Read the model definition and answer for the solid it produces. Units are mm, in the model's axes. A direction names the side the tool comes from. Give positions to 0.01 mm unless a question says otherwise; leave off trailing zeros. Write each loop counter-clockwise with the first axis right and the second up, starting at its lowest first coordinate (ties: lowest second). Pieces come first, ordered by that corner, then holes. Notation, with made-up numbers: (74, 84.25) -> (116, 84.25) arc R21 cw to (116, 112.25) -> close; hole circle Ø7 at (23.5, 67.5). An arc over 180 degrees is marked (long way). Use a Markdown table: item, result.
from build123d import *

# Parameters (mm, degrees)
F0_R      = 6.445170834
F0_R_2    = 6.017003406
F1_DEPTH  = 25.4
F2_W      = 19.7259690613
F2_H      = 52.9098398983
F3_DEPTH  = 25.4
F5_W      = 19.7259690613
F5_H      = 13.0423298106
F6_DEPTH  = 25.4
F4_W      = 19.7259690613
F4_H      = 10.3523302823
F7_DEPTH  = 25.4
F8_R      = 9.8629845306
F9_DEPTH  = 13.208
F12_DEPTH = 10.414
F13_R     = 2.9880803611
F14_DEPTH = 25.4
F15_R     = 2.8379061559
F16_DEPTH = 25.4
F18_DEPTH = 50.8


with BuildPart() as f1:
    # F0 (on Top) → F1 (new body)
    with BuildSketch(Plane.XY):
        with BuildLine():
            Line((23.6895978451, -37.5162102282), (23.6895978451, 37.5162102282))
            ThreePointArc((23.6895978451, 37.5162102282), (0, 61.2058080733), (-23.6895978451, 37.5162102282))
            Line((-23.6895978451, 37.5162102282), (-23.6895978451, -37.5162102282))
            ThreePointArc((-23.6895978451, -37.5162102282), (0, -61.2058080733), (23.6895978451, -37.5162102282))
        make_face()
        with Locations((0, -37.5162102282)):
            Circle(F0_R, mode=Mode.SUBTRACT)
        with Locations((0, 37.5162102282)):
            Circle(F0_R_2, mode=Mode.SUBTRACT)
    extrude(amount=F1_DEPTH)

    # F2 (on face) → F3 (join)
    with BuildSketch(Plane.XY.offset(25.4)):
        Rectangle(F2_W, F2_H)
    extrude(amount=F3_DEPTH)

    # F5 (on face) → F6 (join)
    with BuildSketch(Plane.XY.offset(50.8)):
        with Locations((0, -19.9337550439)):
            Rectangle(F5_W, F5_H)
    extrude(amount=F6_DEPTH)

    # F4 (on face) → F7 (join)
    with BuildSketch(Plane.XY.offset(50.8)):
        with Locations((0, 21.278754808)):
            Rectangle(F4_W, F4_H)
    extrude(amount=F7_DEPTH)

    # F8 (on face) → F9 (join)
    with BuildSketch(Plane.XZ.offset(26.4549199492)):
        with Locations((0, 76.2)):
            Circle(F8_R)
    extrude(amount=-F9_DEPTH)

    # F11 (on face) → F12 (join)
    with BuildSketch(Plane(origin=(0, 26.4549199492, 0), x_dir=(-1, 0, 0), z_dir=(0, 1, 0))):
        with BuildLine():
            Line((-9.8629845306, 76.2), (9.8629845306, 76.2))
            ThreePointArc((9.8629845306, 76.2), (0, 86.0629845306), (-9.8629845306, 76.2))
        make_face()
    extrude(amount=-F12_DEPTH)

    # F13 (on face) → F14 (cut)
    with BuildSketch(Plane.XZ.offset(-16.0409199492)):
        with Locations((-1.1676928261, 80.6610658765)):
            Circle(F13_R)
    extrude(amount=-F14_DEPTH, mode=Mode.SUBTRACT)

    # F15 (on face) → F16 (cut)
    with BuildSketch(Plane(origin=(0, -13.2469199492, 0), x_dir=(-1, 0, 0), z_dir=(0, 1, 0))):
        with Locations((0, 81.546805799)):
            Circle(F15_R)
    extrude(amount=-F16_DEPTH, mode=Mode.SUBTRACT)

    # F17 (on face) → F18 (cut)
    with BuildSketch(Plane(origin=(-9.8629845306, 0, 0), x_dir=(0, -1, 0), z_dir=(-1, 0, 0))):
        with BuildLine():
            ThreePointArc((-16.1025896668, 50.8), (-1.3449997641, 36.0424100973), (13.4125901386, 50.8))
            Line((13.4125901386, 50.8), (-16.1025896668, 50.8))
        make_face()
    extrude(amount=-F18_DEPTH, mode=Mode.SUBTRACT)


solid = f1.part
Item 1: Straight lines are drawn through the part: line 1 along Y through (x, z) = (0, 5.5); line 2 along Y through (x, z) = (0.5, 54); line 3 along Z through (x, y) = (-15.5, -5). For each, find the intervals that lie inside material, in ascending order. Write a range as [from, to].
Return value:
| item | result |
|---|---|
| line 1 | [-61.21, -43.96], [-31.07, 31.5], [43.53, 61.21] |
| line 2 | [-26.45, -13.41], [16.1, 26.45] |
| line 3 | [0, 25.4] |
Item 2: A cutting plane is placed at A-A (z = 59). Give the vertices of the cut face in (x, y), then the cut area to 3 significant figures.
Return value:
| item | result |
|---|---|
| outline | (-9.86, -26.45) -> (9.86, -26.45) -> (9.86, -13.41) -> (-9.86, -13.41) -> close; (-9.86, 16.1) -> (9.86, 16.1) -> (9.86, 26.45) -> (-9.86, 26.45) -> close |
| area | 461 mm^2 |
Item 3: Each of these flat-tipped pins is pushed along its axis until it touches: P1, Ø2, axis at x = 9, y = 9.5, coming from the +Z side; P2, Ø16, axis at x = -0.5, z = 67.5, coming from the -Y side; P3, Ø10, axis at y = -30.5, z = 33.5, coming from the -X side. Where does it stop, or does it pass through?
Return value:
| item | result |
|---|---|
| P1 | z = 39.23 |
| P2 | y = -26.45 |
| P3 | x = -9.86 |
Item 4: A cutting plane is placed at C-C (x = 0). Count the separate pieces of the cut face and the enclosed holes in it, then the cut area to 3 significant figures.
Return value:
| item | result |
|---|---|
| separate pieces | 5 |
| enclosed holes | 0 |
| area | 4,170 mm^2 |
Item 5: A tool of negligible diameter and unlimited length cuts with its end or side. For faces 1 (the face through (9.863, 0, 34)), 2 (the face through (-9.863, 0, 34)), 3 (the face through (-1.557, 21.175, 83.624)), 4 (the face through (0, 26.455, 56)), from which of +Z, -Z, +X, -X, +Y, -Y can it reach the whole face along a straight path? Write none if from no direction.
Return value:
| item | result |
|---|---|
| face 1 | +Z, +X, +Y, -Y |
| face 2 | +Z, -X, +Y, -Y |
| face 3 | +Y |
| face 4 | +Z, +X, -X, +Y |
Item 6: A cutting plane is placed at D-D (z = 11.5). Give the vertices of the cut face in (x, y), then the cut area to 3 significant figures.
Return value:
| item | result |
|---|---|
| outline | (-23.69, -37.52) arc R23.69 ccw to (23.69, -37.52) -> (23.69, 37.52) arc R23.69 ccw to (-23.69, 37.52) -> close; hole circle Ø12.89 at (0, -37.52); hole circle Ø12.03 at (0, 37.52) |
| area | 5,070 mm^2 |
Item 7: For a pull along X with two mould halves and no side action, classify faces 5 (the face through (-1.31, -19.76, 79.03)), 6 (the face through (2, 16.041, 80)), 7 (the face through (2.78, 32.18, 12.52)), 8 (the face through (-0.22, 21.32, 86.06)) as +X half, -X half, draft (parallel to the pull), parting line (faces both ways), or undercut.
Return value:
| item | result |
|---|---|
| face 5 | undercut |
| face 6 | draft |
| face 7 | undercut |
| face 8 | parting line |
Item 8: A cutting plane is placed at B-B (y = -32.5). Give the vertices of the cut face in (x, z).
Return value:
| item | result |
|---|---|
| outline | (-23.69, 0) -> (-4.05, 0) -> (-4.05, 25.4) -> (-23.69, 25.4) -> close; (4.05, 0) -> (23.69, 0) -> (23.69, 25.4) -> (4.05, 25.4) -> close |
